The listing builds one solid part. Answer for the finished solid, in the listing's coordinates (mm). Give positions to 0.01 mm unless a question says otherwise; leave off trailing zeros. Order: outer loops, then holes, each group sorted by start corner. A loop starts at its lowest first (then second) coordinate and runs counter-clockwise, first axis right, second up.
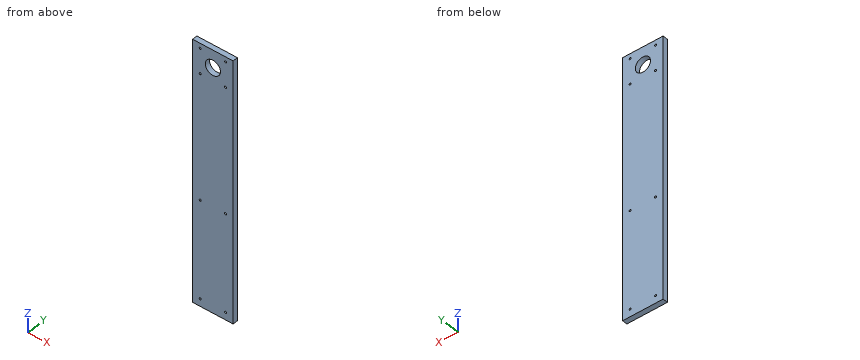
```python
from build123d import *

# Parameters (mm, degrees)
F0_W     = 101.6
F0_H     = 660.4
F0_R     = 2.5527
F0_R_2   = 19.05
F1_DEPTH = 12.7


with BuildPart() as f1:
    # F0 (on Front) → F1 (new body)
    with BuildSketch(Plane.XZ):
        Rectangle(F0_W, F0_H)
        with Locations((-31.75, -311.15)):
            Circle(F0_R, mode=Mode.SUBTRACT)
        with Locations((-31.75, -63.5)):
            Circle(F0_R, mode=Mode.SUBTRACT)
        with Locations((31.75, -311.15)):
            Circle(F0_R, mode=Mode.SUBTRACT)
        with Locations((31.75, -63.5)):
            Circle(F0_R, mode=Mode.SUBTRACT)
        with Locations((-31.75, 254)):
            Circle(F0_R, mode=Mode.SUBTRACT)
        with Locations((-31.75, 317.5)):
            Circle(F0_R, mode=Mode.SUBTRACT)
        with Locations((0, 285.75)):
            Circle(F0_R_2, mode=Mode.SUBTRACT)
        with Locations((31.75, 254)):
            Circle(F0_R, mode=Mode.SUBTRACT)
        with Locations((31.75, 317.5)):
            Circle(F0_R, mode=Mode.SUBTRACT)
    extrude(amount=F1_DEPTH)


solid = f1.part
```
1) Find section A-A (y = -5). Count the separate pieces of the cut face and the enclosed holes in it, then the cut area to 3 significant figures.
Geometry says:
separate pieces: 1
enclosed holes: 9
area: 65,800 mm2
2) Straight lines are drawn through the part: probe 1 along Z at (x, y) = (31.75, -7.5); probe 2 along X at (y, z) = (-4.75, 254); probe 3 along Z at (x, y) = (-32.5, -10). For each, find the intervals that lie inside material, in ascending order.
Geometry says:
probe 1: z = -330.2 to -313.7, -308.6 to -66.05, -60.95 to 251.45, 256.55 to 314.95, 320.05 to 330.2
probe 2: x = -50.8 to -34.3, -29.2 to 29.2, 34.3 to 50.8
probe 3: z = -330.2 to -313.59, -308.71 to -65.94, -61.06 to 251.56, 256.44 to 315.06, 319.94 to 330.2
3) Given P1, Ø4.5, axis at x = -31.75, z = -311.15, coming from the +Y side, flat-ended and moving along its own axis, determine where the tip first touches the part or whether it passes through.
Geometry says:
P1: passes through
4) Find section B-B (x = 0). Write down the section's boundary in (y, z).
Geometry says:
outline: (-12.7, -330.2) - (0, -330.2) - (0, 266.7) - (-12.7, 266.7) - close; (-12.7, 304.8) - (0, 304.8) - (0, 330.2) - (-12.7, 330.2) - close
